Autodesk Inventor part; units mm, degrees
ref_plane "YZ Plane" through (0, 0, 0) normal (1, 0, 0) x (0, 1, 0)
ref_plane "XZ Plane" through (0, 0, 0) normal (0, 1, 0) x (-1, 0, 0)
ref_plane "XY Plane" through (0, 0, 0) normal (0, 0, 1) x (1, 0, 0)
sketch "スケッチ1" plane through (0, 0, 0) normal (0, 1, 0) x (-1, 0, 0)
  line L0 (-10, 12) -> (10, 12)
  line L1 (10, 12) -> (10, -22)
  line L2 (10, -22) -> (-10, -22)
  line L3 (-10, -22) -> (-10, 12)
  circle A0 centre (0, 0) radius 12
  point P0 (10, 6.6332)
  point P1 (-10, 6.6332)
  dimension "d47" = 20
  dimension "d66" = 10
  dimension "d67" = 22
  dimension "d70" = 12
extrude "押し出し1" add sketch "スケッチ1" along normal blind 8 contours A0 L1 L3 | A0 L1 L2 L3
sketch "スケッチ3" plane through (0, 8, 0) normal (0, 1, 0) x (1, 0, 0)
  circle A0 centre (0, 0) radius 8.5
  point P0 (-6.0104, 6.0104)
  point P1 (-6.0104, -6.0104)
  point P2 (6.0104, -6.0104)
  point P3 (6.0104, 6.0104)
  dimension "d6" = 17
  dimension "d9" = 360
hole "穴1" at (-6.0104, 8, -6.0104) at (-6.0104, 8, 6.0104) at (6.0104, 8, 6.0104) at (6.0104, 8, -6.0104) direction (0, -1, 0) diameter 3.2 end through all
sketch "スケッチ2" plane through (0, 8, 0) normal (0, 1, 0) x (1, 0, 0)
  line L0 (-0.5, 0) -> (0.5, 0)
  line L1 (0.5, 0) -> (0.5, 22)
  line L2 (0.5, 22) -> (-0.5, 22)
  line L3 (-0.5, 22) -> (-0.5, 0)
  arc A0 (-10, -6.6332) -> (10, -6.6332) centre (0, 0) ccw
  line L4 (10, 22) -> (-10, 22)
  dimension "d3" = 1
  dimension "d71" = 0.5
extrude "押し出し2" cut sketch "スケッチ2" against normal blind 8
sketch "スケッチ7" plane through (10, 0, 12) normal (1, 0, 0) x (0, 0, -1)
  line L0 (5.3668, 8) -> (34, 8)
  line L1 (34, 0) -> (34, 8)
  line L2 (12, -2) -> (12, 12)
  point P0 (12, 0)
  point P1 (22, 4)
  point P2 (30, 4)
  dimension "d48" = 4
  dimension "d50" = 4
  dimension "d68" = 10
hole "穴4" at (10, 4, -10) at (10, 4, -18) direction (-1, 0, 0) diameter 3.2 end through all
fillet "フィレット1" radius 1 4 edges at (10, 4, -22) (-10, 4, -22) (10, 4, 6.6332) (-10, 4, 6.6332)
sketch "スケッチ8" plane through (0, 0, 0) normal (0, -1, 0) x (1, 0, 0)
  circle A0 centre (0, 0) radius 3
  dimension "d62" = 6
extrude "押し出し4" cut sketch "スケッチ8" against normal through all
chamfer "面取り2" distance 0.5 angle 45 7 edges at (-0.5, 8, -12.479) (0.5, 8, -12.479) (0, 8, 3) (-0.5, 4, -22) (0.5, 4, -22) (0.5, 4, -2.958) (-0.5, 4, -2.958)
properties part number "s_base3"
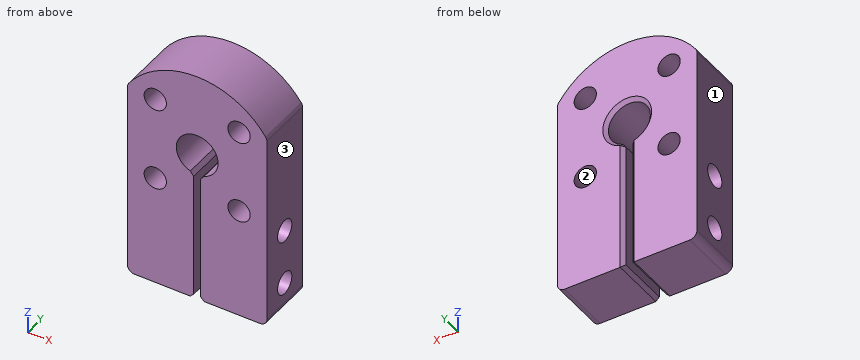
CAD build for the part. Positions are in the model's coordinates, mm. Face numbers are marked on the shaded views. Coordinates: 2 decimals unless noted, no trailing zeros. Write each loop counter-clockwise with the first axis right and the second up, starting at its lowest first coordinate (ties: lowest second). Pieces come first, ordered by that corner, then holes.
(1) Cut at D-D, the plane z = 5. List the corners of the cut face in (x, y), and give its area (3 significant figures).
(2) Drill centre lines: probe 1 along X at (y, z) = (4.25, -15); probe 2 along Z at (x, y) = (2.25, 4.75); probe 3 along Z at (x, y) = (-5.75, 7). Where is each one in solid material? Low to high.
(3) Two-plate mould, pull along X, no slides. Class the marked faces 1, 2 and 3: +X half, -X half, draft (parallel to the pull), parting line (faces both ways), or undercut.
(4) Cut at A-A, the plane z = 0. List the corners of the cut face in (x, y).
(5) Cut at B-B, the plane z = -10. List the corners of the cut face in (x, y).
(6) Cut at C-C, the plane x = 6.5. List the corners of the cut face in (y, z).
Geometry says:
1. outline: (-10, 0) - (-7.25, 0) - (-7.25, 8) - (-10, 8) - close; (-4.77, 0) - (4.77, 0) - (4.77, 8) - (-4.77, 8) - close; (7.25, 0) - (10, 0) - (10, 8) - (7.25, 8) - close
1. area: 120 mm2
2. probe 1: x = -10 to -0.5, 0.5 to 10
2. probe 2: z = -22 to -19.41, -16.59 to -11.41, -8.59 to -1.98, 1.98 to 11.79
2. probe 3: z = -22 to -7.59, -4.43 to 4.43, 7.59 to 10.53
3. face 1: -X half
3. face 2: undercut
3. face 3: +X half
4. outline: (-10, 0) - (-3, 0) - (-3, 7.5) - (-3.5, 8) - (-10, 8) - close; (3, 0) - (10, 0) - (10, 8) - (3.5, 8) - (3, 7.5) - close
5. outline: (-10, 0) - (-0.5, 0) - (-0.5, 2.4) - (-10, 2.4) - close; (-10, 5.6) - (-0.5, 5.6) - (-0.5, 7.5) - (-1, 8) - (-10, 8) - close; (0.5, 0) - (10, 0) - (10, 2.4) - (0.5, 2.4) - close; (0.5, 5.6) - (10, 5.6) - (10, 8) - (1, 8) - (0.5, 7.5) - close
6. outline: (0, -22) - (8, -22) - (8, -7.53) - (0, -7.53) - close; (0, -4.49) - (8, -4.49) - (8, 4.49) - (0, 4.49) - close; (0, 7.53) - (8, 7.53) - (8, 10.09) - (0, 10.09) - close; hole circle Ø3.2 at (4, -18); hole circle Ø3.2 at (4, -10)
